```python
from build123d import *

# Parameters (mm, degrees)
F1_DEPTH = 6.35
F2_SIZE  = 1.016
F3_SIZE  = 1.016


# Not quite as in the source:
# - a feature of the source that left no trace in its solid (it failed there, or was rolled back) is left out


with BuildPart() as f1:
    # F0 (on Front) → F1 (new body)
    with BuildSketch(Plane.XZ):
        Polygon((25.4, 0), (0, 0), (0.0169261405, -6.35), (6.3669261405, -6.35), (6.3669261405, -12.7), (0, -12.7), (0, -19.05), (19.05, -19.05), (19.05, -25.4), (25.4, -25.4), (25.4, -12.7), (19.05, -12.7), (19.05, -6.35), (25.4, -6.35), align=None)
    extrude(amount=F1_DEPTH)

    # F2
    f2_edges = [f1.edges().sort_by_distance(p)[0] for p in [
        (22.225, -6.35, -25.4),
    ]]
    chamfer(f2_edges, length=F2_SIZE)

    # F3
    f3_edges = [f1.edges().sort_by_distance(p)[0] for p in [
        (25.4, -2.667, -25.4),
    ]]
    chamfer(f3_edges, length=F3_SIZE)


solid = f1.part
```
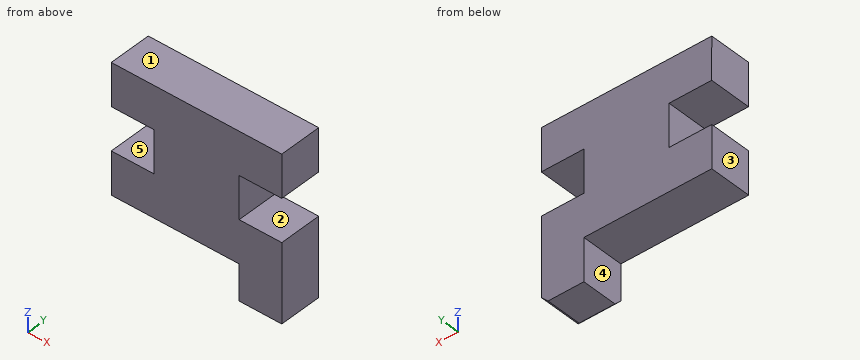
Geometry: final body of the model. Coordinates: model frame, mm. Face numbers are marked on the shaded views. A direction names the side the tool comes from. Coordinates: 2 decimals unless noted, no trailing zeros. Order: outer loops, then holes, each group sorted by start corner. A loop starts at its lowest first (then second) coordinate and runs counter-clockwise, first axis right, second up. Notation, with made-up numbers: (60.5, 3.25) - (105.5, 3.25) arc R21 cw to (105.5, 7.25) - close; hole circle Ø1 at (86, -11). An arc over 180 degrees is marked (long way). Write each question's results on one line, items separated by ' | '.
1) Line query: line 1 (Z direction, x = 4.25, y = -2); line 2 (Z direction, x = 23.5, y = -3.5); line 3 (X direction, y = -0.25, z = -23). Output: solid intervals per line, ascending. Write a range as from..to.
Results list:
line 1: -19.05..-12.7, -6.35..0 | line 2: -25.4..-12.7, -6.35..0 | line 3: 19.05..25.4
2) Section D-D, the plane x = 10.5. Return loops of the section in (y, z).
Results list:
outline: (-6.35, -19.05) - (0, -19.05) - (0, 0) - (-6.35, 0) - close
3) Set-up query: the marked faces 1, 2, 3, 4 and 5. Return all of +Z, -Z, +X, -X, +Y, -Y with unobstructed straight access to the full face (end or side cutting, diameter ignored); none if empty.
Results list:
face 1: +Z, +X, -X, +Y, -Y | face 2: +X, +Y, -Y | face 3: +Z, -Z, -X, +Y, -Y | face 4: -Z, -X, +Y, -Y | face 5: -X, +Y, -Y
4) Section B-B, the plane y = -0.75. Return loops of the section in (x, z), plus the area to 3 significant figures.
Results list:
outline: (0, -19.05) - (19.05, -19.05) - (19.05, -25.4) - (24.38, -25.4) - (25.4, -24.38) - (25.4, -12.7) - (19.05, -12.7) - (19.05, -6.35) - (25.4, -6.35) - (25.4, 0) - (0, 0) - (0.02, -6.35) - (6.37, -6.35) - (6.37, -12.7) - (0, -12.7) - close | area: 443 mm^2
5) Section A-A, the plane x = 21.25. Return loops of the section in (y, z), plus the area to 3 significant figures.
Results list:
outline: (-6.35, -24.38) - (-5.33, -25.4) - (0, -25.4) - (0, -12.7) - (-6.35, -12.7) - close; (-6.35, -6.35) - (0, -6.35) - (0, 0) - (-6.35, 0) - close | area: 120 mm^2
6) Section C-C, the plane x = 4.75. Return loops of the section in (y, z).
Results list:
outline: (-6.35, -19.05) - (0, -19.05) - (0, -12.7) - (-6.35, -12.7) - close; (-6.35, -6.35) - (0, -6.35) - (0, 0) - (-6.35, 0) - close
7) Pin query (flat end, axial travel): pin 1 (1.9 mm diameter, centred on y = -2, z = -10, fed in from -X); pin 2 (1.5 mm diameter, centred on y = -3.5, z = -2.5, fed in from -X); pin 3 (1.9 mm diameter, centred on y = -2.5, z = -23, fed in from -X). Return the tip coordinate at first contact, or that it passes through.
Results list:
pin 1: x = 6.37 | pin 2: x = 0 | pin 3: x = 19.05
